Could you check a few things on this model? Use its own coordinates, in mm. Face numbers are marked on the shaded views. A direction names the side the tool comes from. Coordinates: 2 decimals unless noted, no trailing zeros. Order: outer loops, then holes, each group sorted by start corner. A loop starts at its lowest first (then second) coordinate and runs counter-clockwise, first axis right, second up. Notation, with made-up numbers: (33, -4.5) - (39, -4.5) arc R28 cw to (39, 34.5) - close; hole circle Ø2 at (29, -3.75). An arc over 180 degrees is marked (long way). One line per item, written item: value.
from build123d import *

# Parameters (mm, degrees)
SKETCH1_R           = 35
BOSS_EXTRUDE1_DEPTH = 35
SKETCH2_R           = 35
BOSS_EXTRUDE2_DEPTH = 5
SKETCH7_R           = 7.5
BOSS_EXTRUDE5_DEPTH = 26
CHAMFER1_SIZE       = 2
SKETCH8_R           = 18.7
CUT_EXTRUDE1_DEPTH  = 22
SKETCH11_R          = 30
CUT_EXTRUDE2_DEPTH  = 30


with BuildPart() as part:
    # Sketch1 → Boss-Extrude1 (new body)
    with BuildSketch(Plane.XY):
        Circle(SKETCH1_R)
    extrude(amount=BOSS_EXTRUDE1_DEPTH)

    # Sketch2 → Boss-Extrude2 (add)
    with BuildSketch(Plane.XY.offset(35)):
        Circle(SKETCH2_R)
    extrude(amount=BOSS_EXTRUDE2_DEPTH)

    # Loft1: read off the stored shape, not the designer's step
    # Loft1: loft between two sections, ruled curve by curve
    loft1_from = [
        Edge.make_bspline([(9.456775653, -3.251060481, 0), (2.954654692, -22.164611787, 0), (-15.958896614, -15.662490826, 0), (-9.456775653, 3.251060481, 0), (-2.954654692, 22.164611787, 0), (15.958896614, 15.662490826, 0), (9.456775653, -3.251060481, 0)], [0, 0, 0, 0, 0.5, 0.5, 0.5, 1, 1, 1, 1], 3, [1, 0.333333333, 0.333333333, 1, 0.333333333, 0.333333333, 1]),
    ]
    loft1_to = [
        Edge.make_bspline([(7.055763885, 2.542871605, -7), (12.141507096, -11.568656164, -7), (-1.970020674, -16.654399375, -7), (-7.055763885, -2.542871605, -7), (-12.141507096, 11.568656164, -7), (1.970020674, 16.654399375, -7), (7.055763885, 2.542871605, -7)], [0, 0, 0, 0, 0.5, 0.5, 0.5, 1, 1, 1, 1], 3, [1, 0.333333333, 0.333333333, 1, 0.333333333, 0.333333333, 1]),
    ]
    loft1 = Solid(Shell([*[Face.make_surface_from_curves(loft1_from[k], loft1_to[k]) for k in range(1)], Face(Wire(loft1_from)), Face(Wire(loft1_to))]))
    add(loft1)

    # Sketch7 → Boss-Extrude5 (add)
    with BuildSketch(Plane(origin=(0, 0, -7), x_dir=(-1, 0, 0), z_dir=(0, 0, -1))):
        with Locations(Location((0, 0, 0), (0, 0, 160.181022053))):
            Circle(SKETCH7_R)
    extrude(amount=BOSS_EXTRUDE5_DEPTH)

    # Chamfer1
    chamfer1_edges = [part.edges().sort_by_distance(p)[0] for p in [
        (-7.055763885, -2.542871605, -33),
    ]]
    chamfer(chamfer1_edges, length=CHAMFER1_SIZE)

    # Sketch8 → Cut-Extrude1 (cut)
    with BuildSketch(Plane.XY.offset(40)):
        Circle(SKETCH8_R)
    extrude(amount=-CUT_EXTRUDE1_DEPTH, mode=Mode.SUBTRACT)

    # Sketch11 → Cut-Extrude2 (cut)
    with BuildSketch(Plane.XY.offset(40)):
        Circle(SKETCH11_R)
    extrude(amount=-CUT_EXTRUDE2_DEPTH, mode=Mode.SUBTRACT)


solid = part.part
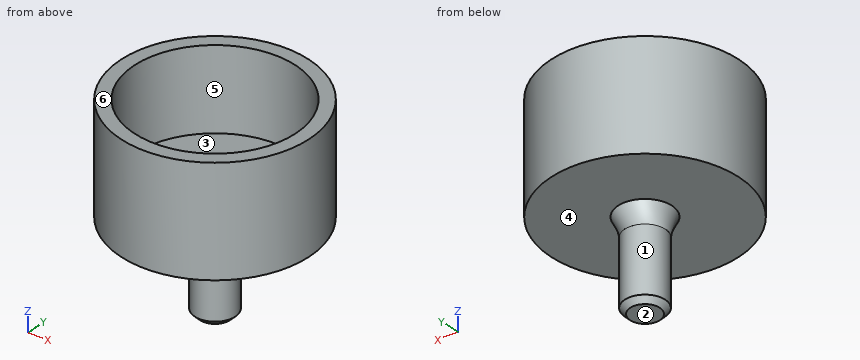
Item 1: I want a section at B-B on z = 11. Please give me the cut outline in (x, y), then the cut area to 3 significant figures.
Conclusion:
outline: circle Ø70 at (0, 0); hole circle Ø60 at (0, 0)
area: 1,020 mm²
Item 2: I'm going to push flat-ended pins straight in: pin 1 Ø6 at (y, z) = (17, 16) entering from +X; pin 2 Ø1.5 at (x, y) = (-18, -0.5) entering from +Z; pin 3 Ø12 at (x, z) = (-21.5, 31) entering from +Y; pin 4 Ø6 at (y, z) = (1.5, 24) entering from -X. Where does each tip first touch, or does it pass through?
Conclusion:
pin 1: x = 32.08
pin 2: z = 10
pin 3: y = 31.38
pin 4: x = -35
Item 3: I want a section at C-C on y = -29. Please give me the cut outline in (x, z).
Conclusion:
outline: (-19.6, 0) - (19.6, 0) - (19.6, 40) - (7.68, 40) - (7.68, 10) - (-7.68, 10) - (-7.68, 40) - (-19.6, 40) - close
Item 4: I want a section at A-A on x = -28. Please give me the cut outline in (y, z), then the cut area to 3 significant figures.
Conclusion:
outline: (-21, 0) - (21, 0) - (21, 40) - (10.77, 40) - (10.77, 10) - (-10.77, 10) - (-10.77, 40) - (-21, 40) - close
area: 1,030 mm²
Item 5: If I drill on probe 1 along Y at (x, z) = (0, 31.75); probe 2 along Z at (x, y) = (27, 10); probe 3 along Z at (x, y) = (-17, -27), over which ranges is the centre line in solid material (lowest first)?
Conclusion:
probe 1: -35 to -30, 30 to 35
probe 2: 0 to 10
probe 3: 0 to 40
Item 6: Thinking about a two-plate mould opening in Y: for the marked faces 1, 2 and 3, which applies, pulls with the +Y half, pulls with the -Y half, needs draft (parallel to the pull), parting line crosses it, or undercut?
Conclusion:
face 1: parting line crosses it
face 2: needs draft
face 3: undercut
Item 7: For the marked faces 4, 5 and 6, which set-ups out of +Z, -Z, +X, -X, +Y, -Y let a thin tool reach every point of the face, with its end or its side?
Conclusion:
face 4: -Z
face 5: +Z
face 6: +Z, +X, -X, +Y, -Y
Item 8: I want a section at D-D on z = -24.5. Please give me the cut outline in (x, y).
Conclusion:
outline: circle Ø15 at (0, 0)
